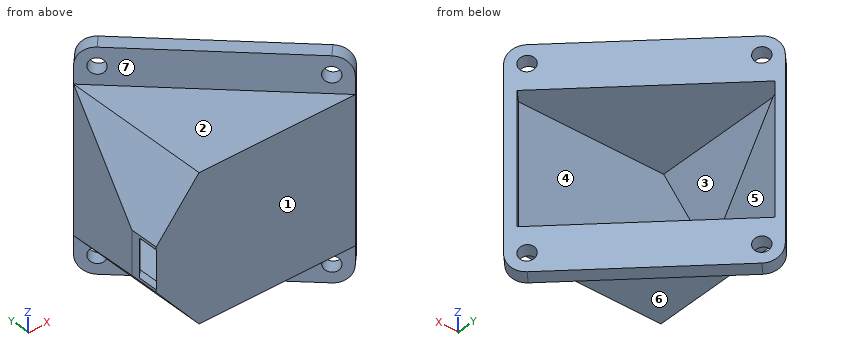
from build123d import *

# Parameters (mm, degrees)
F1_DEPTH = 31.75
F3_DEPTH = 33.8770445158
F4_T     = -1.5875
F5_W     = 3.0979418965
F5_H     = 8.3555914986
F6_DEPTH = 31.3793581519
F7_W     = 47.625
F7_H     = 7.9375
F7_R     = 1.7272
F7_H_2   = 31.75
F7_W_2   = 43.5875253129
F7_H_3   = 28.575
F8_DEPTH = 3.175
F9_R     = 3.96875


with BuildPart() as f1:
    # F0 (on Top) → F1 (new body)
    with BuildSketch(Plane.XY):
        Polygon((-43.9269818101, 0), (0, 0), (-34.4563574527, 32.8770445158), (-43.9269818101, 6.35), align=None)
    extrude(amount=F1_DEPTH)

    # F2 (on face) → F3 (cut, up to face)
    with BuildSketch(Plane.XZ):
        Polygon((-43.9269818101, 11.1125), (-43.9269818101, 0), (-34.4563574527, 0), align=None)
        Polygon((-34.4563574527, 31.75), (-43.9269818101, 31.75), (-43.9269818101, 20.6375), align=None)
    extrude(amount=-F3_DEPTH, mode=Mode.SUBTRACT)

    # F4
    f4_openings = [f1.faces().sort_by_distance(p)[0] for p in [
        (-17.228179, 16.438522, 15.875),
    ]]
    offset(amount=F4_T, openings=f4_openings)

    # F5 (on face) → F6 (cut, up to face)
    with BuildSketch(Plane(origin=(0, 0, 0), x_dir=(-0.7234930699, 0.6903316434, 0), z_dir=(0.6903316434, 0.7234930699, 0))):
        with Locations((33.2771941037, 15.875)):
            Rectangle(F5_W, F5_H)
    extrude(amount=-F6_DEPTH, mode=Mode.SUBTRACT)

    # F7 (on face) → F8 (join)
    with BuildSketch(Plane(origin=(0, 0, 0), x_dir=(-0.7234930699, 0.6903316434, 0), z_dir=(0.6903316434, 0.7234930699, 0))):
        with Locations((23.8125, -3.96875)):
            Rectangle(F7_W, F7_H)
        with Locations((3.96875, -3.96875)):
            Circle(F7_R, mode=Mode.SUBTRACT)
        with Locations((43.65625, -3.96875)):
            Circle(F7_R, mode=Mode.SUBTRACT)
        with Locations((23.8125, 35.71875)):
            Rectangle(F7_W, F7_H)
        with Locations((3.96875, 35.71875)):
            Circle(F7_R, mode=Mode.SUBTRACT)
        with Locations((43.65625, 35.71875)):
            Circle(F7_R, mode=Mode.SUBTRACT)
        with Locations((23.8125, 15.875)):
            Rectangle(F7_W, F7_H_2)
        with Locations((24.0933819992, 15.875)):
            Rectangle(F7_W_2, F7_H_3, mode=Mode.SUBTRACT)
    extrude(amount=F8_DEPTH)

    # F9
    f9_edges = [f1.edges().sort_by_distance(p)[0] for p in [
        (-33.360456, 34.02559, -7.9375),
        (1.095901, 1.148545, -7.9375),
        (-33.360456, 34.02559, 39.6875),
        (1.095901, 1.148545, 39.6875),
    ]]
    fillet(f9_edges, radius=F9_R)


solid = f1.part
Input: part model. Units: mm. Frame: model coordinates. Face numbers are marked on the shaded views. A direction names the side the tool comes from. Coordinates: 2 decimals unless noted, no trailing zeros. Order: outer loops, then holes, each group sorted by start corner. A loop starts at its lowest first (then second) coordinate and runs counter-clockwise, first axis right, second up. Notation, with made-up numbers: M 62,-9.75 L 66,-9.75 A29 cw 66,19.25 Z; hole C -28.75,67 d1. An arc over 180 degrees is marked long. Answer in a Markdown table with one row per item.
(1) Section query D-D, the plane x = -18. Output: boundary loops of the cut face in (y, z), plus the area to 3 significant figures.
Numbers:
| item | result |
|---|---|
| outline | M 0,0 L 17.17,0 L 17.17,-7.94 L 21.56,-7.94 L 21.56,1.59 L 1.59,1.59 L 1.59,30.16 L 21.56,30.16 L 21.56,39.69 L 17.17,39.69 L 17.17,31.75 L 0,31.75 Z |
| area | 183 mm^2 |
(2) Section query B-B, the plane y = 26. Output: boundary loops of the cut face in (x, z), plus the area to 3 significant figures.
Numbers:
| item | result |
|---|---|
| outline | M -36.91,2.88 L -34.46,0 L -27.25,0 L -27.25,-7.94 L -22.65,-7.94 L -22.65,1.59 L -33.72,1.59 L -35.23,3.35 L -35.23,28.4 L -33.72,30.16 L -22.65,30.16 L -22.65,39.69 L -27.25,39.69 L -27.25,31.75 L -34.46,31.75 L -36.91,28.87 Z |
| area | 162 mm^2 |
(3) Section query A-A, the plane z = 14. Output: boundary loops of the cut face in (x, y), plus the area to 3 significant figures.
Numbers:
| item | result |
|---|---|
| outline | M -43.93,4.41 L -42.34,6.08 L -33.2,31.68 L -31.01,33.97 L -32.26,35.17 L -34.46,32.88 L -43.93,6.35 Z; M -43.85,0 L 0,0 L 2.19,2.3 L 0.53,3.88 L -1.66,1.59 L -42.34,1.59 Z |
| area | 125 mm^2 |
(4) Access query for the marked faces 4, 5, 6 and 7. Directions: +Z, -Z, +X, -X, +Y, -Y. A direction counts if a zero-diameter tool reaches every point of the face in a straight line with its end or side. Return the directions, or none.
Numbers:
| item | result |
|---|---|
| face 4 | none |
| face 5 | +X |
| face 6 | -Z, -X, -Y |
| face 7 | +Z, -X, -Y |
(5) Draft query along Z for the marked faces 1, 2 and 3. Return one class per face: pulls with the +Z half, pulls with the -Z half, needs draft (parallel to the pull), parting line crosses it, or undercut.
Numbers:
| item | result |
|---|---|
| face 1 | needs draft |
| face 2 | pulls with the +Z half |
| face 3 | undercut |
(6) Contact query for flat-ended pins moving along their axis: pin 1 Ø1 at (y, z) = (28, 33.5) entering from -X; pin 2 Ø0.8 at (x, y) = (-43.5, 2.5) entering from -Z; pin 3 Ø1.5 at (y, z) = (15, 23.5) entering from -X. Output: stop coordinate, or through.
Numbers:
| item | result |
|---|---|
| pin 1 | stops at x = -29.87 |
| pin 2 | stops at z = 10.14 |
| pin 3 | stops at x = -41.11 |
(7) Section query C-C, the plane z = 24. Output: boundary loops of the cut face in (x, y), plus the area to 3 significant figures.
Numbers:
| item | result |
|---|---|
| outline | M -41.06,0 L 0,0 L 2.19,2.3 L 0.53,3.88 L -1.66,1.59 L -38.98,1.59 L -38.98,15.5 L -33.2,31.68 L -31.01,33.97 L -32.26,35.17 L -34.46,32.88 L -41.06,14.38 Z |
| area | 134 mm^2 |
(8) Material intervals for line 1 (Z direction, x = -16, y = 18.5); line 2 (Z direction, x = -24.5, y = 7.5); line 3 (Y direction, x = -25, z = 19), sorted ascending. Write a range as [from, to].
Numbers:
| item | result |
|---|---|
| line 1 | z = [-7.94, 1.59], [30.16, 39.69] |
| line 2 | z = [0, 1.59], [30.16, 31.75] |
| line 3 | y = [0, 1.59] |
